Read the model definition and answer for the solid it produces. Units are mm, in the model's axes. A direction names the side the tool comes from. Give positions to 0.01 mm unless a question says otherwise; leave off trailing zeros. Order: outer loops, then holes, each group sorted by start corner. A loop starts at its lowest first (then second) coordinate and runs counter-clockwise, first axis right, second up. Notation, with made-up numbers: (34, 24.5) -> (80, 24.5) arc R23 ccw to (80, 32.5) -> close; hole circle Ø7 at (70.5, 79). An arc over 180 degrees is marked (long way). Use one line per item in the form item = value.
```python
from build123d import *

# Parameters (mm, degrees)
SKETCH_R        = 6.5
SKETCH_R_2      = 3
SKETCH_R_3      = 4.5
SKETCH_R_4      = 3.5
PAD_DEPTH       = 8
CHAMFER_SIZE    = 4
CHAMFER001_SIZE = 2.5


with BuildPart() as part:
    # Sketch → Pad (new body)
    with BuildSketch(Plane.XY):
        with BuildLine():
            Line((223, 0), (576, 0))
            ThreePointArc((576, 0), (607.819805, 13.180195), (621, 45))
            Line((621, 45), (621, 128))
            ThreePointArc((633, 140), (624.514719, 136.485281), (621, 128))
            Line((633, 140), (796, 140))
            ThreePointArc((800, 136), (798.828427, 138.828427), (796, 140))
            Line((800, -96), (800, 136))
            ThreePointArc((796, -100), (798.828427, -98.828427), (800, -96))
            Line((796, -100), (-786, -100))
            ThreePointArc((-790, -96), (-788.828427, -98.828427), (-786, -100))
            Line((-790, 136), (-790, -96))
            ThreePointArc((-786, 140), (-788.828427, 138.828427), (-790, 136))
            Line((-786, 140), (-412, 140))
            ThreePointArc((-362.763287, 125.337548), (-386.313226, 136.256534), (-412, 140))
            Line((-362.763287, 125.337548), (-311.236713, 91.662452))
            ThreePointArc((-311.236713, 91.662452), (-287.686774, 80.743466), (-262, 77))
            Line((-262, 77), (158, 77))
            ThreePointArc((178, 57), (172.142136, 71.142136), (158, 77))
            Line((178, 57), (178, 45))
            ThreePointArc((178, 45), (191.180195, 13.180195), (223, 0))
        make_face()
        with Locations((-715, 50)):
            Circle(SKETCH_R, mode=Mode.SUBTRACT)
        with Locations((-665, 33)):
            Circle(SKETCH_R, mode=Mode.SUBTRACT)
        with Locations((-715, -26)):
            Circle(SKETCH_R, mode=Mode.SUBTRACT)
        with Locations((-307.5, -26)):
            Circle(SKETCH_R, mode=Mode.SUBTRACT)
        with Locations((-307.5, -74)):
            Circle(SKETCH_R, mode=Mode.SUBTRACT)
        with Locations((0, -74)):
            Circle(SKETCH_R, mode=Mode.SUBTRACT)
        with Locations((0, -26)):
            Circle(SKETCH_R, mode=Mode.SUBTRACT)
        with Locations((307.5, -74)):
            Circle(SKETCH_R, mode=Mode.SUBTRACT)
        with Locations((307.5, -26)):
            Circle(SKETCH_R, mode=Mode.SUBTRACT)
        with Locations((715, -26)):
            Circle(SKETCH_R, mode=Mode.SUBTRACT)
        with Locations((715, -74)):
            Circle(SKETCH_R, mode=Mode.SUBTRACT)
        with Locations((307.5, -50)):
            Circle(SKETCH_R_2, mode=Mode.SUBTRACT)
        with Locations((-307.5, -50)):
            Circle(SKETCH_R_2, mode=Mode.SUBTRACT)
        with Locations((-715, -74)):
            Circle(SKETCH_R, mode=Mode.SUBTRACT)
        with Locations((-430, 130)):
            Circle(SKETCH_R_2, mode=Mode.SUBTRACT)
        with Locations((-430, 71)):
            Circle(SKETCH_R_2, mode=Mode.SUBTRACT)
        with Locations((615, -26)):
            Circle(SKETCH_R, mode=Mode.SUBTRACT)
        with Locations((665, -26)):
            Circle(SKETCH_R, mode=Mode.SUBTRACT)
        with Locations((615, -74)):
            Circle(SKETCH_R, mode=Mode.SUBTRACT)
        with Locations((665, -74)):
            Circle(SKETCH_R, mode=Mode.SUBTRACT)
        with Locations((0, -50)):
            Circle(SKETCH_R_2, mode=Mode.SUBTRACT)
        with Locations((790, -50)):
            Circle(SKETCH_R_2, mode=Mode.SUBTRACT)
        with Locations((742, 125)):
            Circle(SKETCH_R, mode=Mode.SUBTRACT)
        with Locations((765, 113)):
            Circle(SKETCH_R, mode=Mode.SUBTRACT)
        with Locations((765, 87)):
            Circle(SKETCH_R, mode=Mode.SUBTRACT)
        with Locations((742, 75)):
            Circle(SKETCH_R, mode=Mode.SUBTRACT)
        with Locations((-665, -74)):
            Circle(SKETCH_R, mode=Mode.SUBTRACT)
        with Locations((-615, -74)):
            Circle(SKETCH_R, mode=Mode.SUBTRACT)
        with Locations((-665, -26)):
            Circle(SKETCH_R, mode=Mode.SUBTRACT)
        with Locations((-615, -26)):
            Circle(SKETCH_R, mode=Mode.SUBTRACT)
        with Locations((-396.782, 53.2)):
            Circle(SKETCH_R_3, mode=Mode.SUBTRACT)
        with Locations((5.218, 53.2)):
            Circle(SKETCH_R_3, mode=Mode.SUBTRACT)
        with Locations((45.218, 53.2)):
            Circle(SKETCH_R_3, mode=Mode.SUBTRACT)
        with Locations((85.218, 53.2)):
            Circle(SKETCH_R_3, mode=Mode.SUBTRACT)
        with Locations((125.218, 53.2)):
            Circle(SKETCH_R_3, mode=Mode.SUBTRACT)
        with Locations((790, 10)):
            Circle(SKETCH_R_2, mode=Mode.SUBTRACT)
        with Locations((790, 130)):
            Circle(SKETCH_R_2, mode=Mode.SUBTRACT)
        with Locations((-740, -50)):
            Circle(SKETCH_R_2, mode=Mode.SUBTRACT)
        with Locations((-740, 10)):
            Circle(SKETCH_R_4, mode=Mode.SUBTRACT)
        with Locations((-740, 130)):
            Circle(SKETCH_R_2, mode=Mode.SUBTRACT)
        with Locations((387.5, -26)):
            Circle(SKETCH_R, mode=Mode.SUBTRACT)
        with Locations((467.5, -26)):
            Circle(SKETCH_R, mode=Mode.SUBTRACT)
        with Locations((547.5, -26)):
            Circle(SKETCH_R, mode=Mode.SUBTRACT)
        with Locations((158, 62)):
            Circle(SKETCH_R_2, mode=Mode.SUBTRACT)
        with Locations((158, 10)):
            Circle(SKETCH_R_2, mode=Mode.SUBTRACT)
        with Locations((-770, -74)):
            Circle(SKETCH_R, mode=Mode.SUBTRACT)
        with Locations((-770, 114)):
            Circle(SKETCH_R, mode=Mode.SUBTRACT)
        with Locations((-740, 30)):
            Circle(SKETCH_R_2, mode=Mode.SUBTRACT)
        with Locations((-770, 20)):
            Circle(SKETCH_R, mode=Mode.SUBTRACT)
        with Locations((-405, 125)):
            Circle(SKETCH_R_3, mode=Mode.SUBTRACT)
        with Locations((688.8, 30)):
            Circle(SKETCH_R, mode=Mode.SUBTRACT)
        with Locations((-265.282, 71)):
            Circle(SKETCH_R_4, mode=Mode.SUBTRACT)
        with Locations((-215.282, 71)):
            Circle(SKETCH_R_4, mode=Mode.SUBTRACT)
        with Locations((615, -50)):
            Circle(SKETCH_R_2, mode=Mode.SUBTRACT)
        with Locations((-615, -50)):
            Circle(SKETCH_R_2, mode=Mode.SUBTRACT)
        with BuildLine():
            ThreePointArc((-690, 85), (-675, 100), (-690, 115))
            ThreePointArc((-690, 115), (-705, 100), (-690, 85))
        make_face(mode=Mode.SUBTRACT)
        with BuildLine():
            Line((688.243823, 120.3), (689.056177, 120.3))
            ThreePointArc((689.056177, 120.3), (690.950364, 120.561153), (692.703215, 121.325126))
            ThreePointArc((702.325126, 111.703215), (701.3, 120.3), (692.703215, 121.325126))
            ThreePointArc((702.325126, 111.703215), (701.561153, 109.950364), (701.3, 108.056177))
            Line((701.3, 108.056177), (701.3, 91.943823))
            ThreePointArc((701.3, 91.943823), (701.561153, 90.049636), (702.325126, 88.296785))
            ThreePointArc((692.703215, 78.674874), (701.3, 79.7), (702.325126, 88.296785))
            ThreePointArc((692.703215, 78.674874), (690.950364, 79.438847), (689.056177, 79.7))
            Line((689.056177, 79.7), (688.243823, 79.7))
            ThreePointArc((688.243823, 79.7), (686.349636, 79.438847), (684.596785, 78.674874))
            ThreePointArc((674.974874, 88.296785), (676, 79.7), (684.596785, 78.674874))
            ThreePointArc((674.974874, 88.296785), (675.738847, 90.049636), (676, 91.943823))
            Line((676, 91.943823), (676, 108.056177))
            ThreePointArc((676, 108.056177), (675.738847, 109.950364), (674.974874, 111.703215))
            ThreePointArc((684.596785, 121.325126), (676, 120.3), (674.974874, 111.703215))
            ThreePointArc((684.596785, 121.325126), (686.349636, 120.561153), (688.243823, 120.3))
        make_face(mode=Mode.SUBTRACT)
        with BuildLine():
            Line((738.898235, 106.2), (745.101765, 106.2))
            ThreePointArc((745.101765, 106.2), (745.642961, 106.274615), (746.143776, 106.492893))
            ThreePointArc((748.892893, 103.743776), (748.6, 106.2), (746.143776, 106.492893))
            ThreePointArc((748.892893, 103.743776), (748.674615, 103.242961), (748.6, 102.701765))
            Line((748.6, 102.701765), (748.6, 97.298235))
            ThreePointArc((748.6, 97.298235), (748.674615, 96.757039), (748.892893, 96.256224))
            ThreePointArc((746.143776, 93.507107), (748.6, 93.8), (748.892893, 96.256224))
            ThreePointArc((746.143776, 93.507107), (745.642961, 93.725385), (745.101765, 93.8))
            Line((745.101765, 93.8), (738.898235, 93.8))
            ThreePointArc((738.898235, 93.8), (738.357039, 93.725385), (737.856224, 93.507107))
            ThreePointArc((735.107107, 96.256224), (735.4, 93.8), (737.856224, 93.507107))
            ThreePointArc((735.107107, 96.256224), (735.325385, 96.757039), (735.4, 97.298235))
            Line((735.4, 97.298235), (735.4, 102.701765))
            ThreePointArc((735.4, 102.701765), (735.325385, 103.242961), (735.107107, 103.743776))
            ThreePointArc((737.856224, 106.492893), (735.4, 106.2), (735.107107, 103.743776))
            ThreePointArc((737.856224, 106.492893), (738.357039, 106.274615), (738.898235, 106.2))
        make_face(mode=Mode.SUBTRACT)
    extrude(amount=PAD_DEPTH)

    # Chamfer
    chamfer_edges = [part.edges().sort_by_distance(p)[0] for p in [
        (-3, -50, 0),
        (-310.5, -50, 0),
        (155, 10, 0),
        (-743, 30, 0),
        (-618, -50, 0),
        (-743, 130, 0),
        (-743, -50, 0),
        (612, -50, 0),
        (155, 62, 0),
        (304.5, -50, 0),
    ]]
    chamfer(chamfer_edges, length=CHAMFER_SIZE)

    # Chamfer001
    chamfer001_edges = [part.edges().sort_by_distance(p)[0] for p in [
        (-743.5, 10, 8),
    ]]
    chamfer(chamfer001_edges, length=CHAMFER001_SIZE)


solid = part.part
```
Item 1: Given pin 1 Ø8 at (x, y) = (-665, 33) entering from +Z; pin 2 Ø2.5 at (x, z) = (321.5, 5) entering from +Y; pin 3 Ø3 at (x, z) = (16.5, 4) entering from +Y, each flat-ended and moving along its own axis, determine where each tip first touches the part or whether it passes through.
Checks:
pin_1 = through
pin_2 = 0
pin_3 = 77
Item 2: Determine the mould class of faces 1 (the flat face through (16, -5, 8)), 2 (the cylindrical face through (-675.357, 96.748, 3.944)), 3 (the cylindrical face through (607.468, 12.832, 3.944)) for opening direction X: +X half, -X half, draft (parallel to the pull), parting line (faces both ways), or undercut.
Checks:
face_1 = draft
face_2 = undercut
face_3 = undercut
Item 3: The part is cut by section B-B on x = 414. Give the vertices of the cut face in (y, z), and give its area (3 significant figures).
Checks:
outline = (-100, 0) -> (0, 0) -> (0, 8) -> (-100, 8) -> close
area = 800 mm²
Item 4: Which of the six approach directions +Z, -Z, +X, -X, +Y, -Y give full straight-line access (tool end or side, diameter ignored) to faces 4 (the flat face through (-337.361, 108.736, 3.944)), 5 (the flat face through (16, -5, 0))?
Checks:
face_4 = +Z, -Z, +Y
face_5 = -Z, +X, -X, +Y, -Y
Item 5: Straight lines are drawn through the part: L1, parallel to Y at x = 715, z = 5.25; L2, parallel to Y at x = 790, z = 6; L3, parallel to X at y = 48, z = 1.5. For each, find the intervals that lie inside material, in ascending order. Write a range as from..to.
Checks:
L1 = -100..-80.5, -67.5..-32.5, -19.5..140
L2 = -100..-53, -47..7, 13..127, 133..140
L3 = -790..-721.18, -708.82..178, 621..800
Item 6: The part is cut by section C-C on x = -70. Give the vertices of the cut face in (y, z).
Checks:
outline = (-100, 0) -> (77, 0) -> (77, 8) -> (-100, 8) -> close
Item 7: The part is cut by section A-A on z = 6.75. State how many separate pieces and enclosed holes the cut face has, and give its area (3 significant figures).
Checks:
separate_pieces = 1
enclosed_holes = 58
area = 281,000 mm²
